Autodesk Fusion 360 part; units mm, degrees
sketch "Sketch1" plane through (0, 0, 0) normal (0, 0, 1) x (1, 0, 0)
  circle A0 centre (0, 0) radius 20
  dimension "d1" = 40
extrude "Extrude1" add sketch "Sketch1" along normal blind 150 makes body 1
sketch "Sketch2" plane through (0, 0, 0) normal (0, 1, 0) x (1, 0, 0)
  line L0 (-20, 0) -> (20, 0) construction
  line L1 (-20, -150) -> (20, -150) construction
  line L2 (0, -150) -> (0, 0) construction
  line L3 (-20, -150) -> (-20, 0) construction
  line L4 (-20, 0) -> (-35.25, 0)
  line L5 (-35.25, 0) -> (-35.25, -15.25)
  line L6 (-35.25, -15.25) -> (-20, -15.25)
  line L7 (-27.625, -15.25) -> (-27.625, 0) construction
  circle A0 centre (-27.625, -7.625) radius 2.625
  circle A1 centre (-27.625, -7.625) radius 1.5
  line L8 (-20, -15.25) -> (0, -15.25)
  line L9 (-20, 0) -> (0, 0)
  line L10 (20, -15.25) -> (0, -15.25)
  line L11 (35.25, -15.25) -> (20, -15.25)
  line L12 (35.25, 0) -> (35.25, -15.25)
  line L13 (20, 0) -> (35.25, 0)
  line L14 (20, 0) -> (0, 0)
  circle A2 centre (27.625, -7.625) radius 2.625
  circle A3 centre (27.625, -7.625) radius 1.5
  line L15 (20, -15.25) -> (20, 0)
  line L16 (-20, -15.25) -> (-20, 0)
  line L17 (20, -15.25) -> (20, 0)
  line L18 (-20, -15.25) -> (-20, 0)
  point P0 (-27.625, -7.625)
  dimension "d5" = 5.25
  dimension "d6" = 3
  dimension "d7" = 5
  dimension "d8" = 5
  dimension "d13" = 5
ref_plane "WorkPlane1" through (0, -20, 103.4458) normal (0, -1, 0) x (-1, 0, 0)
extrude "Extrude2" add sketch "Sketch2" against normal blind 55 from surface at -20 separate body contours L4 L5 L6 L16 L18 | L8 L9 L10 L14 L15 L16 L17 L18 | L11 L12 L13 L15 L17 | A0 | A2 makes body 2
extrude "Extrude3" add sketch "Sketch2" along normal blind 20 from surface at -20 contours L8 L9 L10 L14 L15 L16 L17 L18 bodies 1 2
move_face "OffsetFaces1" offset -50 2 faces at (27.6624, -20, 13.2069) (-27.5876, -20, 13.2069) on bodies 1
extrude "Extrude4" cut sketch "Sketch2" against normal blind 2.5 from surface at -70 contours A0 | A2 bodies 1
fillet "Fillet1" radius 5 4 edges at (35.25, -72.5, 15.25) (35.25, -72.5, 0) (-35.25, -72.5, 15.25) (-35.25, -72.5, 0) on bodies 1
sketch "Sketch3" plane through (0, 0, 15.25) normal (0, 0, 1) x (-1, 0, 0)
  line L0 (30.25, 70) -> (30.25, 75)
  line L1 (30.25, 75) -> (-30.25, 75)
  line L2 (-30.25, 75) -> (-30.25, 70)
  line L3 (-30.25, 70) -> (-20, 70)
  line L4 (-20, 70) -> (-20, 0)
  arc A0 (20, 0) -> (-20, 0) centre (0, 0) ccw
  line L5 (20, 0) -> (20, 70)
  line L6 (20, 70) -> (30.25, 70)
  line L7 (-30.25, 75) -> (30.25, 75)
  line L8 (20, 70) -> (20, 0)
  line L9 (-20, 70) -> (-20, 0)
  circle A1 centre (0, 0) radius 20
  line L10 (0, 75) -> (0, 20) construction
  line L11 (17, 23) -> (-17, 23)
  line L12 (-17, 23) -> (-17, 65)
  line L13 (-17, 65) -> (17, 65)
  line L14 (17, 65) -> (17, 23)
  circle A2 centre (0, 0) radius 17.5
  line L15 (-1.5, 65) -> (-1.5, 23)
  line L16 (1.5, 65) -> (1.5, 23)
  dimension "d23" = 3
  dimension "d24" = 3
  dimension "d25" = 5
  dimension "d26" = 3
  dimension "d31" = -2.5
  dimension "d41" = 1.5
extrude "Extrude5" cut sketch "Sketch3" against normal up to surface (15.25 mm away) contours L11 L13 L14 L16 | L11 L12 L13 L15 bodies 1
fillet "Fillet2" radius 5 4 edges at (-17, -65, 7.625) (-17, -23, 7.625) (17, -23, 7.625) (17, -65, 7.625) on bodies 1
extrude "Extrude6" cut sketch "Sketch3" against normal up to surface (150 mm away) from surface at 134.75 contours A2 bodies 1
sketch "Sketch4" plane through (20, 0, 0) normal (1, 0, 0) x (0, 1, 0)
  line L0 (-70, 15.25) -> (-70, 0)
  line L1 (-70, 0) -> (0, 0)
  line L2 (0, 0) -> (0, 15.25)
  line L3 (0, 15.25) -> (-70, 15.25)
  line L4 (-66, 4) -> (-4, 4)
  line L5 (-4, 4) -> (-4, 11.25)
  line L6 (-4, 11.25) -> (-66, 11.25)
  line L7 (-66, 11.25) -> (-66, 4)
  line L8 (0, 15.25) -> (-20, 15.25)
  line L9 (-20, 15.25) -> (-20, 0) construction
  line L10 (-24, 15.25) -> (-24, 0)
  dimension "d35" = -4
  dimension "d36" = 4
Build history of the part. All positions in model axes, mm. A direction names the side the tool comes from. Give positions to 0.01 mm unless a question says otherwise; leave off trailing zeros. Loops run counter-clockwise (first coordinate to the right, second up) from the corner with the lowest first, then second, coordinate; pieces in that order, holes last.
1) Band-saw the part on B-B on y = -15. List the corners of the cut face in (x, z).
Values follow:
outline: (-20, 0) - (-9.01, 0) - (-9.01, 150) - (-13.23, 150) - (-13.23, 15.25) - (-20, 15.25) - close; (9.01, 0) - (20, 0) - (20, 15.25) - (13.23, 15.25) - (13.23, 150) - (9.01, 150) - close
2) Probe line 1 along X through (y, z) = (1, 54.5); line 2 along Y through (x, z) = (0.5, 109); line 3 along Y through (x, z) = (12, 53). List the from-to ranges inside material, lowest first.
Values follow:
line 1: x = -19.97 to -17.47, 17.47 to 19.97
line 2: y = -19.99 to -17.49, 17.49 to 19.99
line 3: y = -16 to -12.74, 12.74 to 16
3) Drop flat-ended pins along their axis: P1, Ø7.5, axis at y = -45.5, z = 5.5, coming from the -X side; P2, Ø12, axis at x = 27.5, z = 6, coming from the +Y side; P3, Ø12, axis at y = -23.5, z = 6.5, coming from the +X side; P4, Ø2.5, axis at x = -27.625, z = 7.625, coming from the +Y side. Give the stop position or say it passes through.
Values follow:
P1: stops at x = -20
P2: stops at y = -70
P3: stops at x = 20
P4: passes through
4) 3-axis set-ups, long thin cutter, end or side, ignore diameter. For faces 4 (the face through (7, -65, 8)), 5 (the face through (25.69, -71.23, 5.85)), 6 (the face through (-24, -70, 8)): which of +Z, -Z, +X, -X, +Y, -Y reach the whole face in a straight line?
Values follow:
face 4: +Z, -Z
face 5: +Y
face 6: +Z, -Z, -X, +Y
5) Band-saw the part on D-D on x = -23. List the corners of the cut face in (y, z).
Values follow:
outline: (-75, 0) - (-70, 0) - (-70, 15.25) - (-75, 15.25) - close
6) Band-saw the part on C-C on z = 36.5. List the corners of the cut face in (x, y).
Values follow:
outline: circle Ø40 at (0, 0); hole circle Ø35 at (0, 0)
7) Band-saw the part on A-A on y = -38. List the corners of the cut face in (x, z), then the cut area to 3 significant figures.
Values follow:
outline: (-20, 0) - (-17, 0) - (-17, 15.25) - (-20, 15.25) - close; (-1.5, 0) - (1.5, 0) - (1.5, 15.25) - (-1.5, 15.25) - close; (17, 0) - (20, 0) - (20, 15.25) - (17, 15.25) - close
area: 137 mm2
8) Two-plate mould, pull along Y, no slides. Class faces 1 (the face through (-4.336, 19.524, 73.95)), 2 (the face through (0, -18, 150)), 3 (the face through (7, -23, 8)): released by +Y, released by -Y, zero draft, split by the parting line, or undercut.
Values follow:
face 1: split by the parting line
face 2: zero draft
face 3: undercut
